Read the model definition and answer for the solid it produces. Units are mm, in the model's axes. Give positions to 0.01 mm unless a question says otherwise; leave off trailing zeros. Order: outer loops, then holes, each group sorted by start corner. A loop starts at its lowest first (then second) coordinate and runs counter-clockwise, first axis right, second up. Notation, with made-up numbers: M -2.75,65 L 18.25,65 A11 cw 18.25,85 Z; hole C -9,76.25 d1. An arc over 180 degrees is marked long. One line per item, written item: value.
from build123d import *

# Parameters (mm, degrees)
F0_R     = 6.35
F1_DEPTH = 25.4
F2_R     = 5.08


with BuildPart() as f1:
    # F0 (on Right) → F1 (new body)
    with BuildSketch(Plane.YZ):
        with BuildLine():
            ThreePointArc((-12.7, 0), (0, 12.7), (12.7, 0))
            Line((12.7, 0), (25.4, 0))
            Line((25.4, 0), (25.4, 15.24))
            Line((25.4, 15.24), (-25.4, 15.24))
            Line((-25.4, 15.24), (-25.4, 0))
            Line((-25.4, 0), (-12.7, 0))
        make_face()
        with BuildLine():
            ThreePointArc((-12.7, 0), (0, -12.7), (12.7, 0))
            ThreePointArc((12.7, 0), (0, 12.7), (-12.7, 0))
        make_face()
        Circle(F0_R, mode=Mode.SUBTRACT)
    extrude(amount=F1_DEPTH)

    # F2
    f2_edges = [f1.edges().sort_by_distance(p)[0] for p in [
        (12.7, -12.7, 0),
        (12.7, 12.7, 0),
        (12.7, 25.4, 0),
        (12.7, -25.4, 0),
    ]]
    fillet(f2_edges, radius=F2_R)


solid = f1.part
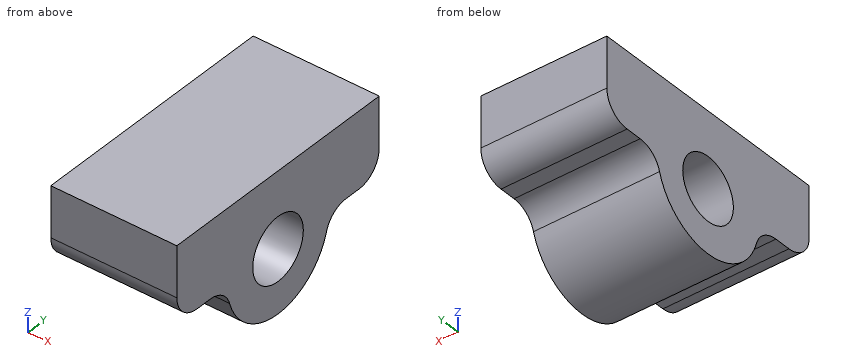
1) Find section A-A, the plane y = 0. Write down the section's boundary in (x, z), plus the area to 3 significant figures.
Reported:
outline: M 0,-12.7 L 25.4,-12.7 L 25.4,-6.35 L 0,-6.35 Z; M 0,6.35 L 25.4,6.35 L 25.4,15.24 L 0,15.24 Z
area: 387 mm^2
2) Each of these flat-tipped pins is pushed along its axis until it touches: pin 1 Ø2 at (x, z) = (12, 0) entering from -Y; pin 2 Ø3 at (x, y) = (7.5, 9) entering from -Z; pin 3 Ø6 at (x, z) = (22, -9.5) entering from +Y. Where does it stop, or does it pass through?
Reported:
pin 1: stops at y = -23.35
pin 2: stops at z = -10.25
pin 3: stops at y = 10.91
3) Find section C-C, the plane z = 2. Write down the section's boundary in (x, y).
Reported:
outline: M 0,-24.36 L 25.4,-24.36 L 25.4,-6.03 L 0,-6.03 Z; M 0,6.03 L 25.4,6.03 L 25.4,24.36 L 0,24.36 Z
4) Find section D-D, the plane y = 16. Write down the section's boundary in (x, z).
Reported:
outline: M 0,-0.11 L 25.4,-0.11 L 25.4,15.24 L 0,15.24 Z
5) Consider probe 1 along Z at (x, y) = (8.5, 1.5); probe 2 along Z at (x, y) = (5.75, 3.5); probe 3 along Y at (x, z) = (4.75, -1.75). Determine where each line is inside the solid, lowest interval first.
Reported:
probe 1: z = -12.61 to -6.17, 6.17 to 15.24
probe 2: z = -12.21 to -5.3, 5.3 to 15.24
probe 3: y = -13.2 to -6.1, 6.1 to 13.2
6) Find section B-B, the plane x = 7. Write down the section's boundary in (y, z), plus the area to 3 significant figures.
Reported:
outline: M -25.4,5.08 A5.08 ccw -20.32,0 L -17.04,0 A5.08 cw -12.17,-3.63 A12.7 ccw 12.17,-3.63 A5.08 cw 17.04,0 L 20.32,0 A5.08 ccw 25.4,5.08 L 25.4,15.24 L -25.4,15.24 Z; hole C 0,0 d12.7
area: 897 mm^2
